Autodesk Inventor part; units mm, degrees
ref_plane "YZ Plane" through (0, 0, 0) normal (1, 0, 0) x (0, 1, 0)
ref_plane "XZ Plane" through (0, 0, 0) normal (0, 1, 0) x (-1, 0, 0)
ref_plane "XY Plane" through (0, 0, 0) normal (0, 0, 1) x (1, 0, 0)
sketch "Sketch1" plane through (0, 0, 0) normal (1, 0, 0) x (0, 1, 0)
  line L0 (-15.875, 19.05) -> (-15.875, -19.05)
  line L1 (-15.875, -19.05) -> (15.875, -19.05)
  line L2 (15.875, -19.05) -> (15.875, 19.05)
  line L3 (15.875, 19.05) -> (-15.875, 19.05)
  line L4 (-15.875, 19.05) -> (15.875, -19.05) construction
  line L5 (-15.875, -19.05) -> (15.875, 19.05) construction
  point P0 (0, 0)
  dimension "d0" = 31.75
  dimension "d1" = 38.1
extrude "Extrusion1" add sketch "Sketch1" against normal blind 6.35
sketch "Sketch2" plane through (0, 0, 0) normal (1, 0, 0) x (0, 0, -1)
  line L0 (-19.05, -15.875) -> (-19.05, 15.875)
  line L1 (19.05, -15.875) -> (-19.05, -15.875)
  line L2 (-19.05, 15.875) -> (-12.7, 15.875)
  line L3 (-12.7, 15.875) -> (-12.7, -15.875)
  line L4 (-12.7, -15.875) -> (-19.05, -15.875)
  line L5 (-19.05, -15.875) -> (-19.05, 15.875)
  point P0 (0, 0)
  dimension "d4" = 6.35
extrude "Extrusion2" add sketch "Sketch2" along normal blind 25.4
sketch "Sketch3" plane through (-6.35, -15.875, 19.05) normal (0, 0, 1) x (1, 0, 0)
  circle A0 centre (18.8501, 15.875) radius 9.525
  line L0 (0, 0) -> (0, 31.75)
  line L1 (31.75, 31.75) -> (31.75, 0) construction
  line L2 (31.75, 15.875) -> (0, 15.875) construction
  line L3 (0, 31.75) -> (0, 0) construction
  point P0 (6.35, 15.875)
  dimension "d7" = 18.8501
  dimension "d8" = 19.05
  dimension "d11" = 0
extrude "Extrusion3" cut sketch "Sketch3" against normal through all
sketch "Sketch4" plane through (0, 0, 0) normal (1, 0, 0) x (0, 0, -1)
  line L0 (9.525, 6.35) -> (-3.175, 6.35) construction
  line L1 (-3.175, 6.35) -> (-3.175, -6.35) construction
  line L2 (-3.175, -6.35) -> (9.525, -6.35) construction
  line L3 (9.525, -6.35) -> (9.525, 6.35) construction
  line L4 (19.05, 15.875) -> (-12.7, 15.875)
  line L5 (19.05, -15.875) -> (19.05, 15.875)
  line L6 (-12.7, -15.875) -> (-12.7, 15.875)
  line L7 (-12.7, -15.875) -> (19.05, -15.875)
  point P0 (0, 0)
  dimension "d12" = 9.525
  dimension "d13" = 9.525
  dimension "d14" = 9.525
  dimension "d15" = 9.525
hole "Hole1" at (0, 6.35, 3.175) at (0, 6.35, -9.525) at (0, -6.35, -9.525) at (0, -6.35, 3.175) direction (-1, 0, 0) diameter 6.7564 end through all
properties part number "sideSupport"
For this review, take the finished solid that the model builds, in its own axes (mm). A direction names the side the tool comes from. Give positions to 0.01 mm unless a question says otherwise; leave off trailing zeros. Loops run counter-clockwise (first coordinate to the right, second up) from the corner with the lowest first, then second, coordinate; pieces in that order, holes last.
Item 1: For line 1 along Z through (x, y) = (-1.25, -6.35); line 2 along Y through (x, z) = (-3, -11) (3 decimals); line 3 along Y through (x, z) = (-1.5, 4) (3 decimals), list the stretches that pass through material, from the lowest coordinate up.
Item 2: Take a section at A-A, the plane y = 0. State the section outline as (x, z) points, and give its area (3 significant figures).
Item 3: Tool access review of faces 1 (the flat face through (13, -10, 12.7)), 2 (the cylindrical face through (-3.22, -6.5, -6.15)): name each direction out of +Z, -Z, +X, -X, +Y, -Y from which nothing blocks a thin tool from reaching the whole face with its end or side.
Item 4: Take a section at D-D, the plane y = 6.35. State the section outline as (x, z) points, and give its area (3 significant figures).
Item 5: Draft analysis for pull direction Y (two halves, no side actions). For faces 3 (the cylindrical face through (-3.22, -7.36, -0.05)), 4 (the flat face through (0, 0, -3)), 5 (the cylindrical face through (-3.22, 5.34, -0.05)), 6 (the flat face through (-1, -15.875, 9)), state which applies: +Y half, -Y half, draft (parallel to the pull), parting line (faces both ways), or undercut.
Item 6: Take a section at B-B, the plane x = 6.5. State the section outline as (y, z) points (3 decimals), and give its area (3 significant figures).
Item 7: Take a section at C-C, the plane x = -2.5. State the section outline as (y, z) points (3 decimals).
Item 8: Insertion check: pin 1 (5 mm diameter, centred on y = 12, z = -2, fed in from +X); pin 2 (4 mm diameter, centred on y = -6.35, z = -9.525, fed in from +X); pin 3 (4 mm diameter, centred on x = 22, y = -1, fed in from -Z). Each pin has a flat end and moves straight along its axis. Give the tip position at first contact, or say it passes through.
Calculated:
1. line 1: z = -19.05 to -12.9, -6.15 to -0.2, 6.55 to 19.05
1. line 2: y = -15.875 to -9.389, -3.311 to 3.311, 9.389 to 15.875
1. line 3: y = -15.875 to -9.626, -3.074 to 3.074, 9.626 to 15.875
2. outline: (-6.35, -19.05) - (0, -19.05) - (0, 12.7) - (2.98, 12.7) - (2.98, 19.05) - (-6.35, 19.05) - close; (22.03, 12.7) - (25.4, 12.7) - (25.4, 19.05) - (22.03, 19.05) - close
2. area: 282 mm2
3. face 1: -Z, +X, +Y, -Y
3. face 2: +X, -X
4. outline: (-6.35, -19.05) - (0, -19.05) - (0, -12.9) - (-6.35, -12.9) - close; (-6.35, -6.15) - (0, -6.15) - (0, -0.2) - (-6.35, -0.2) - close; (-6.35, 6.55) - (0, 6.55) - (0, 12.7) - (5.4, 12.7) - (5.4, 19.05) - (-6.35, 19.05) - close; (19.6, 12.7) - (25.4, 12.7) - (25.4, 19.05) - (19.6, 19.05) - close
4. area: 227 mm2
5. face 3: undercut
5. face 4: draft
5. face 5: undercut
5. face 6: -Y half
6. outline: (-15.875, 12.7) - (-7.398, 12.7) - (-7.398, 19.05) - (-15.875, 19.05) - close; (7.398, 12.7) - (15.875, 12.7) - (15.875, 19.05) - (7.398, 19.05) - close
6. area: 108 mm2
7. outline: (-15.875, -19.05) - (15.875, -19.05) - (15.875, 19.05) - (-15.875, 19.05) - close; hole circle Ø6.756 at (-6.35, -9.525); hole circle Ø6.756 at (-6.35, 3.175); hole circle Ø6.756 at (6.35, -9.525); hole circle Ø6.756 at (6.35, 3.175)
8. pin 1: stops at x = 0
8. pin 2: passes through
8. pin 3: stops at z = 12.7
